Part model, mm, in its own coordinate system. Face numbers are marked on the shaded views. Give positions to 0.01 mm unless a question says otherwise; leave off trailing zeros. Order: outer loops, then holes, each group sorted by start corner. A loop starts at its lowest first (then second) coordinate and runs counter-clockwise, first axis right, second up. Notation, with made-up numbers: M -36.5,86.5 L -9.5,86.5 A19 cw -9.5,121.5 Z; hole C 6,56.25 d2. An arc over 180 degrees is marked long. Return JSON: item names as keys, results as strings.
Autodesk Inventor part; units mm, degrees
ref_plane "YZ Plane" through (0, 0, 0) normal (1, 0, 0) x (0, 1, 0)
ref_plane "XZ Plane" through (0, 0, 0) normal (0, 1, 0) x (-1, 0, 0)
ref_plane "XY Plane" through (0, 0, 0) normal (0, 0, 1) x (1, 0, 0)
sketch "Sketch4" plane through (0, 0, 0) normal (0, 0, 1) x (1, 0, 0)
  line L0 (0, 0) -> (-30, 0)
  line L1 (-30, 0) -> (-30, 40)
  line L2 (-30, 40) -> (0, 40)
  line L3 (0, 40) -> (0, 0)
  dimension "d37" = 30
  dimension "d38" = 40
extrude "Extrusion2" add sketch "Sketch4" along normal blind 14
hole "Hole3" at (-22.5, 35, 14) direction (0, 0, -1) diameter 4.134 depth 14.2 tip angle 118
hole "Hole4" at (-7.5, 35, 14) direction (0, 0, -1) diameter 4.134 depth 14.2 tip angle 118
hole "Hole5" at (-7.5, 5, 14) direction (0, 0, -1) diameter 4.134 depth 14.2 tip angle 118
hole "Hole6" at (-22.5, 5, 14) direction (0, 0, -1) diameter 4.134 depth 14.2 tip angle 118
hole "Hole7" at (0, 20, -1) direction (-1, 0, 0) diameter 22 end through all
fillet "Fillet1" radius 5 4 edges at (-30, 40, 7) (0, 40, 7) (0, 0, 7) (-30, 0, 7)
properties part number "GARFO" material "Aluminium AW-7020"
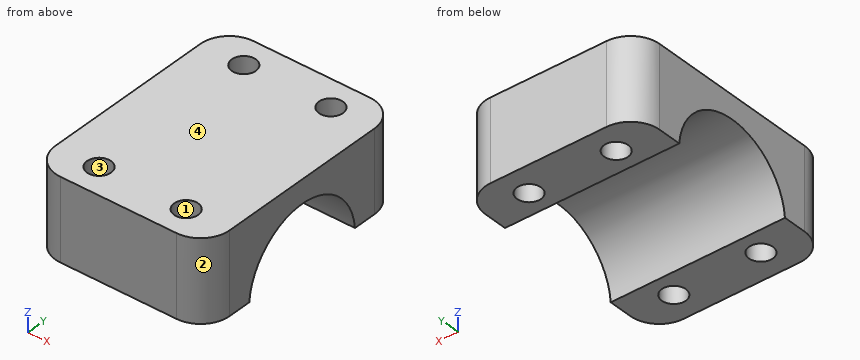
Q1. Band-saw the part on A-A (z = 6.5). Give the cut face in (x, y).
Established:
{"outline": "M -30,5 A5 ccw -25,0 L -5,0 A5 ccw 0,5 L 0,11.95 L -30,11.95 Z; M -30,28.05 L 0,28.05 L 0,35 A5 ccw -5,40 L -25,40 A5 ccw -30,35 Z; hole C -22.5,5 d4.13; hole C -22.5,35 d4.13; hole C -7.5,5 d4.13; hole C -7.5,35 d4.13"}
Q2. Band-saw the part on D-D (x = -15.5). Give the cut face in (y, z), then the cut area to 3 significant figures.
Established:
{"outline": "M 0,0 L 9.05,0 A11 cw 30.95,0 L 40,0 L 40,14 L 0,14 Z", "area": "392 mm²"}
Q3. Probe line 1 along X through (y, z) = (5, 10); line 2 along Y through (x, z) = (-7.5, 10.5); line 3 along Y through (x, z) = (-22.5, 5.25). List the from-to ranges inside material, lowest first.
Established:
{"line 1": "x = -30 to -24.57, -20.43 to -9.57, -5.43 to 0", "line 2": "y = 0 to 2.93, 7.07 to 32.93, 37.07 to 40", "line 3": "y = 0 to 2.93, 7.07 to 10.95, 29.05 to 32.93, 37.07 to 40"}
Q4. Band-saw the part on B-B (x = -22.5). Give the cut face in (y, z), then the cut area to 3 significant figures.
Established:
{"outline": "M 0,0 L 2.93,0 L 2.93,14 L 0,14 Z; M 7.07,0 L 9.05,0 A11 cw 30.95,0 L 32.93,0 L 32.93,14 L 7.07,14 Z; M 37.07,0 L 40,0 L 40,14 L 37.07,14 Z", "area": "276 mm²"}
Q5. Two-plate mould, pull along X, no slides. Class the marked faces 1, 2, 3 and 4: +X half, -X half, draft (parallel to the pull), parting line (faces both ways), or undercut.
Established:
{"face 1": "undercut", "face 2": "+X half", "face 3": "undercut", "face 4": "draft"}
Q6. Band-saw the part on C-C (z = 12). Give the cut face in (x, y).
Established:
{"outline": "M -30,5 A5 ccw -25,0 L -5,0 A5 ccw 0,5 L 0,35 A5 ccw -5,40 L -25,40 A5 ccw -30,35 Z; hole C -22.5,5 d4.13; hole C -22.5,35 d4.13; hole C -7.5,5 d4.13; hole C -7.5,35 d4.13"}
Q7. Pin check, flat tip, straight feed: pin 1 (2.5 mm diameter, centred on x = -7.5, y = 35, fed in from -Z). Stop position of the tip, or through.
Established:
{"pin 1": "passes through"}
